Part print with two shaded views. Sizes in mm from the minimum x, y, z corner. A direction names the side the tool comes from. Give positions to 0.01 mm unless a question says otherwise; leave off trailing zeros. Order: outer loops, then holes, each group sorted by start corner. A loop starts at its lowest first (then second) coordinate and runs counter-clockwise, first axis right, second up. Notation, with made-up numbers: (81, -23) -> (131, -23) arc R19 ccw to (131, -10) -> close; hole circle Ø1 at (32, 11). An arc over 180 degrees is marked (long way). Answer as CSV lines item,"result".
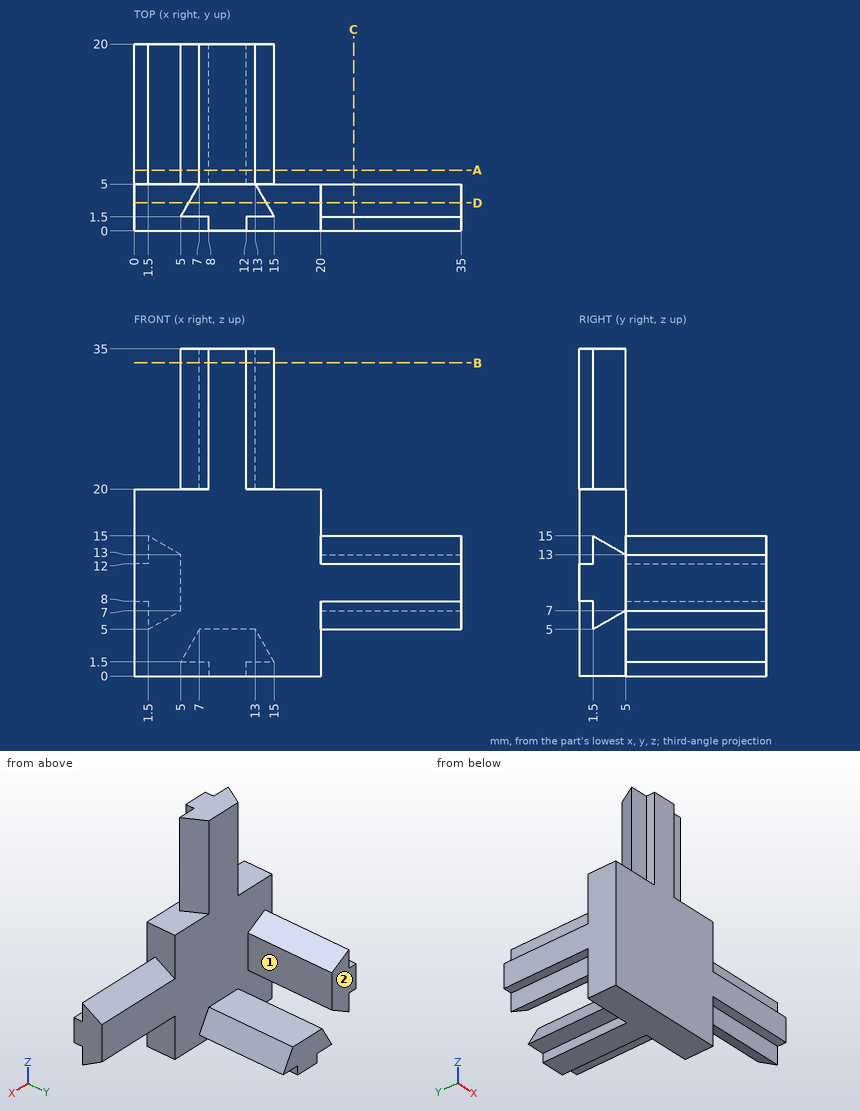
1) Band-saw the part on D-D, the plane y = 3. Write the cut outline in (x, z), then the cut area to 3 significant figures.
Data:
outline,"(0, 0) -> (20, 0) -> (20, 5.86) -> (35, 5.86) -> (35, 14.14) -> (20, 14.14) -> (20, 20) -> (14.14, 20) -> (14.14, 35) -> (5.86, 35) -> (5.86, 20) -> (0, 20) -> close"
area,"649 mm2"
2) Band-saw the part on A-A, the plane y = 6.5. Write the cut outline in (x, z), then the cut area to 3 significant figures.
Data:
outline,"(0, 8) -> (1.5, 8) -> (1.5, 5) -> (5, 7) -> (5, 13) -> (1.5, 15) -> (1.5, 12) -> (0, 12) -> close; (5, 1.5) -> (8, 1.5) -> (8, 0) -> (12, 0) -> (12, 1.5) -> (15, 1.5) -> (13, 5) -> (7, 5) -> close"
area,"68.0 mm2"
3) Pin check, flat tips, straight feed: P1, Ø1, axis at x = 28, z = 14, coming from the +Y side (3 decimals); P2, Ø0.8, axis at x = 24.5, y = 0.5, coming from the -Z side; P3, Ø1.2, axis at x = 24.5, y = 0.5, coming from the +Z side. Stop position of each tip, or through.
Data:
P1,"stops at y = 4.125"
P2,"stops at z = 8"
P3,"stops at z = 12"
4) Which spindle directions (+Z, -Z, +X, -X, +Y, -Y) get a long thin tool onto all of the face, cutting with end or side? Do the marked faces 1 and 2. Say none if no direction does.
Data:
face 1,"+Z, +X, +Y"
face 2,"+Z, -Z, +X, -X, +Y"
5) Band-saw the part on C-C, the plane x = 23.5. Write the cut outline in (y, z).
Data:
outline,"(0, 8) -> (1.5, 8) -> (1.5, 5) -> (5, 7) -> (5, 13) -> (1.5, 15) -> (1.5, 12) -> (0, 12) -> close"
6) Wall check: line 1 along Y through (x, z) = (7.5, 10.5); line 2 along Y through (x, z) = (13.5, 26) (3 decimals). Give the ranges that are in metal, low to high. Write a range as [from, to].
Data:
line 1,"y = [0, 5]"
line 2,"y = [1.5, 4.125]"
7) Band-saw the part on B-B, the plane z = 33.5. Write the cut outline in (x, y).
Data:
outline,"(5, 1.5) -> (8, 1.5) -> (8, 0) -> (12, 0) -> (12, 1.5) -> (15, 1.5) -> (13, 5) -> (7, 5) -> close"
